For this review, use the dimensioned drawing (mm, ordinates from the lowest corner) and the shaded views. A direction names the side the tool comes from. Give positions to 0.01 mm unless a question says otherwise; leave off trailing zeros. Loops run counter-clockwise (first coordinate to the right, second up) from the corner with the lowest first, then second, coordinate; pieces in that order, holes last. Notation, with made-up numbers: (-32.75, 32) - (-8.75, 32) arc R21 ccw to (-8.75, 39) - close; hole circle Ø5 at (84.25, -27). An arc over 180 degrees is marked (long way). Write each question's results on one line, items separated by ' | '.
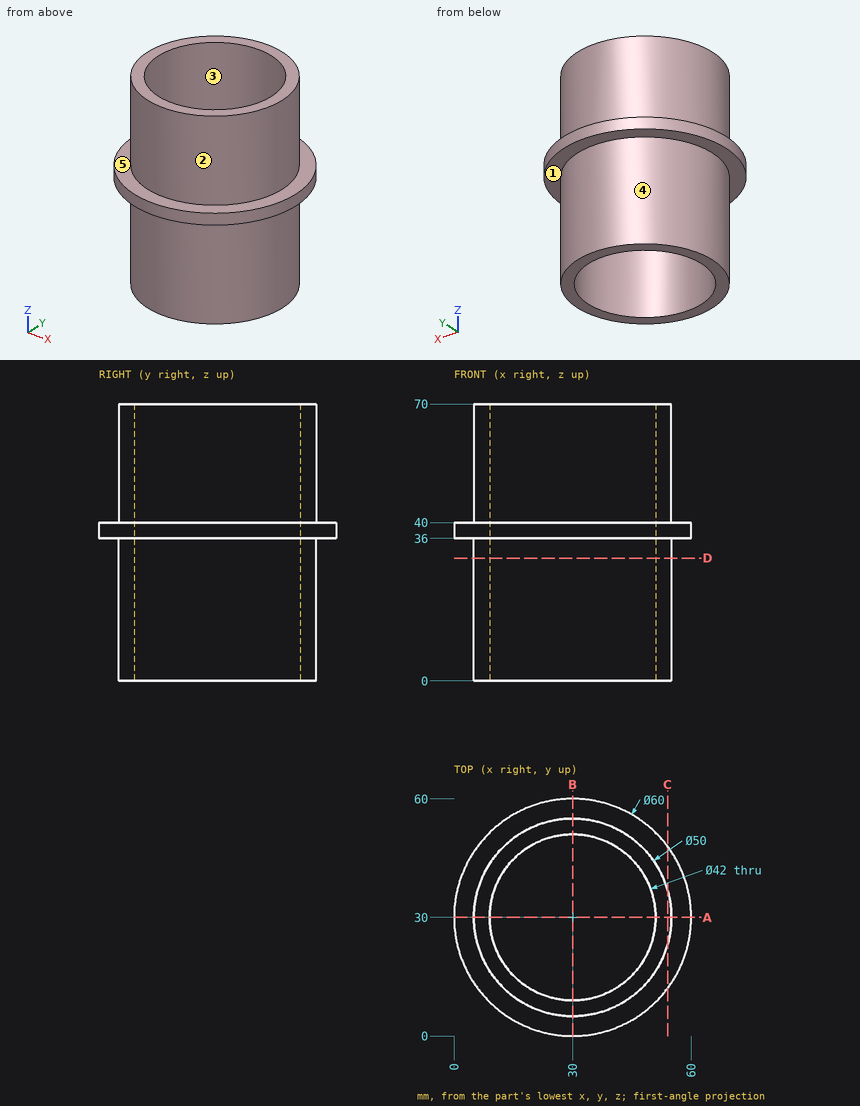
Item 1: We need section A-A on y = 30. Give the boundary of the cut face in (x, z), then the cut area to 3 significant figures.
Output values:
outline: (0, 36) - (5, 36) - (5, 0) - (9, 0) - (9, 70) - (5, 70) - (5, 40) - (0, 40) - close; (51, 0) - (55, 0) - (55, 36) - (60, 36) - (60, 40) - (55, 40) - (55, 70) - (51, 70) - close | area: 600 mm²
Item 2: Clearance check with flat-ended pins moving along their axes: P1, Ø10, axis at y = 51.5, z = 48.5, coming from the -X side; P2, Ø6, axis at x = 24, z = 27.5, coming from the -Y side; P3, Ø10, axis at y = 14, z = 58, coming from the -X side. State where each tip first meets the part, or that it passes through.
Output values:
P1: stops at x = 11.22 | P2: stops at y = 5.18 | P3: stops at x = 7.55
Item 3: Tool access review of the marked faces 4 and 5: name each direction out of +Z, -Z, +X, -X, +Y, -Y from which nothing blocks a thin tool from reaching the whole face with its end or side.
Output values:
face 4: -Z | face 5: +Z
Item 4: Wall thickness on probe 1 along X at (y, z) = (30, 22.5); probe 2 along Y at (x, z) = (24, 47): over which ranges is each line inside the solid? List them lowest first.
Output values:
probe 1: x = 5 to 9, 51 to 55 | probe 2: y = 5.73 to 9.88, 50.12 to 54.27
Item 5: Draft analysis for pull direction Y (two halves, no side actions). For the marked faces 1, 2 and 3, state which applies: +Y half, -Y half, draft (parallel to the pull), parting line (faces both ways), or undercut.
Output values:
face 1: draft | face 2: parting line | face 3: undercut
Item 6: We need section D-D on z = 31. Give the boundary of the cut face in (x, y).
Output values:
outline: circle Ø50 at (30, 30); hole circle Ø42 at (30, 30)
Item 7: We need section C-C on x = 54. Give the boundary of the cut face in (y, z), then the cut area to 3 significant figures.
Output values:
outline: (12, 36) - (23, 36) - (23, 0) - (37, 0) - (37, 36) - (48, 36) - (48, 40) - (37, 40) - (37, 70) - (23, 70) - (23, 40) - (12, 40) - close | area: 1,070 mm²
